Work out the finished part from the listing and answer in its coordinate system (mm). A direction names the side the tool comes from. Round coordinates to 2 decimals unless told otherwise and drop trailing zeros. Loops run counter-clockwise (first coordinate to the right, second up) from the corner with the lowest first, then second, coordinate; pieces in that order, holes last.
from build123d import *

# Parameters (mm, degrees)
F2_R = 1.905


with BuildPart() as f3:
    # F3: sweep along a path in F0
    with BuildLine(Plane.XZ) as f3_path:
        Line((-9.9292984232, 0), (-13.6707741767, 0))
        Line((-13.6707741767, 0), (-13.6707741767, 39.2854884267))
        Line((-13.6707741767, 39.2854884267), (11.6561325267, 39.2854884267))
        Line((11.6561325267, 39.2854884267), (11.6561325267, 0))
        Line((11.6561325267, 0), (8.2024643198, 0))
    # F2 (on offset) → F3 (sweep)
    with BuildSketch(Plane.YZ.offset(-10.033)):
        Circle(F2_R)
    sweep(path=f3_path.line, transition=Transition.RIGHT)


solid = f3.part
Item 1: Section C-C, the plane x = -13.25 is taken. Give the vertices of the cut face in (y, z) (3 decimals), plus the area to 3 significant figures.
Item 2: Section B-B, the plane y = 0 is taken. Give the vertices of the cut face in (x, z) (3 decimals).
Item 3: For faces 1 (the face through (-15.56, -0.25, 19.94)), 2 (the face through (8.202, 0, 0)), determine the directions among +Z, -Z, +X, -X, +Y, -Y from which every point of the face is accessible in a straight line to the end or side of a thin tool.
Item 4: Each of these flat-tipped pins is pushed along its axis until it touches: P1, Ø1, axis at x = 1.5, y = -1.5, coming from the -Z side; P2, Ø3, axis at x = 8.5, z = 25.5, coming from the +Y side; P3, Ø2, axis at x = -2, y = 1, coming from the -Z side. Where does it stop, or does it pass through?
Item 5: Straight lines are drawn through the part: line 1 (Z direction, x = 3.5, y = 0.2); line 2 (X direction, y = -0.1, z = 6); line 3 (X direction, y = 1.4, z = 22.5). For each, find the intervals that lie inside material, in ascending order.
Item 6: Determine the mould class of faces 3 (the face through (10.25, -0.25, -1.89)), 4 (the face through (-9.929, 0, 0)) for opening direction X: pulls with the +X half, pulls with the -X half, needs draft (parallel to the pull), parting line crosses it, or undercut.
Item 7: Section D-D, the plane z = 5 is taken. Give the vertices of the cut face in (x, y) (3 decimals).
Item 8: Section A-A, the plane z = 0 is taken. Give the vertices of the cut face in (x, y) (3 decimals).
Answer below:
1. outline: (-1.858, 0.421) arc R1.905 ccw (long way) to (1.858, 0.421) - (1.858, 38.865) arc R1.905 ccw (long way) to (-1.858, 38.865) - close
1. area: 157 mm2
2. outline: (-15.576, -1.905) - (-9.929, -1.905) - (-9.929, 1.905) - (-11.766, 1.905) - (-11.766, 37.38) - (9.751, 37.38) - (9.751, 1.905) - (8.202, 1.905) - (8.202, -1.905) - (13.561, -1.905) - (13.561, 41.19) - (-15.576, 41.19) - close
3. face 1: none
3. face 2: -Z, +Y, -Y
4. P1: stops at z = 37.66
4. P2: stops at y = 0.94
4. P3: stops at z = 37.38
5. line 1: z = 37.39 to 41.18
5. line 2: x = -15.57 to -11.77, 9.75 to 13.56
5. line 3: x = -14.96 to -12.38, 10.36 to 12.95
6. face 3: undercut
6. face 4: undercut
7. outline: circle Ø3.81 at (-13.671, 0); circle Ø3.81 at (11.656, 0)
8. outline: (-13.671, -1.905) - (-9.929, -1.905) - (-9.929, 1.905) - (-13.671, 1.905) arc R1.905 ccw to start; (8.202, -1.905) - (11.656, -1.905) arc R1.905 ccw to (11.656, 1.905) - (8.202, 1.905) - close
